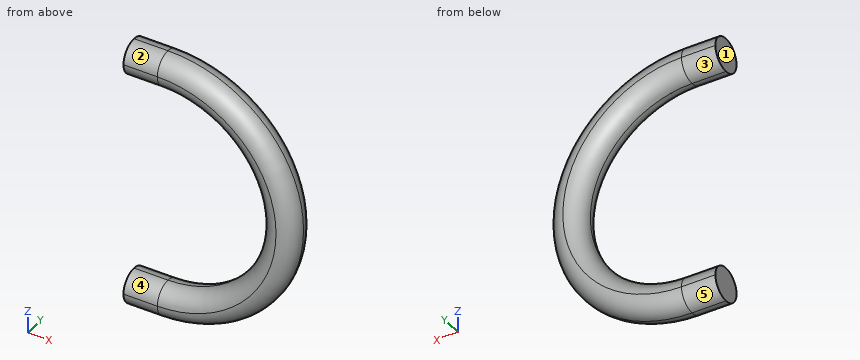
from build123d import *

# Parameters (mm, degrees)
F1_DEPTH = 6.35
F2_R     = 3.17499


# Not quite as in the source:
# - a fillet or chamfer is up to 0.001 mm smaller than in the source, because OpenCascade refuses the exact size


with BuildPart() as f1:
    # F0 (on Front) → F1 (new body)
    with BuildSketch(Plane.XZ):
        with BuildLine():
            Line((0, 6.350000307), (0, 0))
            Line((0, 0), (6.35, 0))
            ThreePointArc((6.35, 0), (31.75, 25.4), (6.35, 50.8))
            Line((6.35, 50.8), (0, 50.8))
            Line((0, 50.8), (0, 44.449999693))
            Line((0, 44.449999693), (6.35, 44.449999693))
            ThreePointArc((6.35, 44.449999693), (25.399999693, 25.4), (6.35, 6.350000307))
            Line((6.35, 6.350000307), (0, 6.350000307))
        make_face()
    extrude(amount=F1_DEPTH)

    # F2 (radius 3.175 in the source; OpenCascade refuses exactly that, so slightly less here)
    f2_edges = [f1.edges().sort_by_distance(p)[0] for p in [
        (31.75, -6.35, 25.4),
        (25.4, -6.35, 25.4),
        (31.75, 0, 25.4),
        (3.175, 0, 6.35),
    ]]
    fillet(f2_edges, radius=F2_R)


solid = f1.part
Work out the finished part from the listing and answer in its coordinate system (mm). Face numbers are marked on the shaded views. A direction names the side the tool comes from. Round coordinates to 2 decimals unless told otherwise and drop trailing zeros. Order: outer loops, then holes, each group sorted by start corner. A loop starts at its lowest first (then second) coordinate and runs counter-clockwise, first axis right, second up. Notation, with made-up numbers: M -32.5,-6.75 L -6.5,-6.75 A10 ccw -6.5,2.25 Z; hole C -24.5,56 d4. An arc over 180 degrees is marked long. Put each result on its own line as item: value. Start each with the question number.
Q1. Section A-A, the plane y = -2.5 is taken. Write down the section's boundary in (x, z).
Q2. Straight lines are drawn through the part: L1, parallel to Z at x = 22, y = -5; L2, parallel to Z at x = 5.5, y = -1.25; L3, parallel to X at y = -0.75, z = 17. For each, find the intervals that lie inside material, in ascending order. Write a range as [from, to].
Q3. For a pull along Z with two mould halves and no side action, classify the marked faces 1, 2 and 3 as pulls with the +Z half, pulls with the -Z half, needs draft (parallel to the pull), parting line crosses it, or undercut.
Q4. Section B-B, the plane y = -5.5 is taken. Write down the section's boundary in (x, z).
Q5. Flat-ended cylindrical pins translate along their axes: pin 1 (2 mm diameter, centred on x = 24, z = 18, fed in from +Y); pin 2 (3 mm diameter, centred on y = -2, z = 10.5, fed in from -X). Find the tip coordinate at first contact, or state that the pin passes through.
Q6. A tool of negligible diameter and unlimited length cuts with its end or side. For the marked faces 4 and 5, from which of +Z, -Z, +X, -X, +Y, -Y can it reach the whole face along a straight path? Write none if from no direction.
Findings below:
1. outline: M 0,0.07 L 6.35,0.07 A25.33 ccw 6.35,50.73 L 0,50.73 L 0,44.52 L 6.35,44.52 A19.12 cw 6.35,6.28 L 0,6.28 Z
2. L1: z = [6.13, 13.56], [37.24, 44.67]
2. L2: z = [0.65, 5.7], [45.1, 50.15]
2. L3: x = [24.69, 29.12]
3. face 1: needs draft
3. face 2: pulls with the +Z half
3. face 3: undercut
4. outline: M 0,1.01 L 6.35,1.01 A24.39 ccw 6.35,49.79 L 0,49.79 L 0,45.46 L 6.35,45.46 A20.06 cw 6.35,5.34 L 0,5.34 Z
5. pin 1: stops at y = -0.78
5. pin 2: stops at x = 16.32
6. face 4: -X, -Y
6. face 5: -Z, +X, -X, +Y
